Could you check a few things on this model? Use its own coordinates, in mm. Face numbers are marked on the shaded views. A direction names the side the tool comes from. Round coordinates to 2 decimals unless told otherwise and drop trailing zeros. Order: outer loops, then holes, each group sorted by start corner. A loop starts at its lowest first (then second) coordinate and runs counter-clockwise, first axis right, second up.
```python
from build123d import *

# Parameters (mm, degrees)
F2_R = 0.25
F3_R = 0.5
F4_R = 0.25


with BuildPart() as f1:
    # F0 (on Right) → F1 (revolve)
    with BuildSketch(Plane.YZ):
        Polygon((4, 6.35), (2.5, 6.35), (2.5, -2.5), (3.7, -2.5), (3.7, 0), (5.42, 0), (5.42, 2), (4, 2), align=None)
    revolve(axis=Axis((0, 0, -1.722812), (0, 0, -1)))

    # F2
    f2_edges = [f1.edges().sort_by_distance(p)[0] for p in [
        (0, -2.5, 6.35),
    ]]
    fillet(f2_edges, radius=F2_R)

    # F3
    f3_edges = [f1.edges().sort_by_distance(p)[0] for p in [
        (0, -4, 6.35),
    ]]
    fillet(f3_edges, radius=F3_R)

    # F4
    f4_edges = [f1.edges().sort_by_distance(p)[0] for p in [
        (0, -5.42, 2),
    ]]
    fillet(f4_edges, radius=F4_R)


solid = f1.part
```
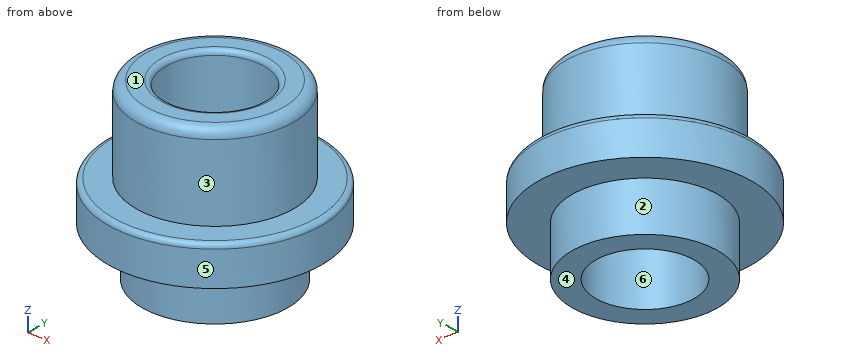
Q1. I need wall thicknesses on L1, parallel to X at y = 0, z = 4.25; L2, parallel to X at y = 0, z = 0.25; L3, parallel to Z at x = -1, y = -4.5. Which ranges of each line are inside material? Lowest first, please.
Q2. We'd pull the mould along Y, two halves only. Please class the marked faces 4, 5 and 6: released by +Y, released by -Y, zero draft, split by the parting line, or undercut.
Q3. Imagine slicing it at A-A, the plane x = 0. Please give me the cut outline in (y, z).
Q4. For P1, Ø6.5, axis at x = 0, y = 0, coming from the +Z side; P2, Ø4, axis at x = -3.5, z = 5, coming from the +Y side; P3, Ø4, axis at x = -4, z = 4.5, coming from the -Y side; P4, Ø1, axis at x = -3, z = 4, coming from the +Y side, each with a flat end and sliding along its axis, tell me the tip position at first contact or that it passes through.
Q5. Imagine slicing it at C-C, the plane z = 0.75. Please give me the cut outline in (x, y), then the cut area to 3 significant figures.
Q6. Imagine slicing it at D-D, the plane z = 3. Please give me the cut outline in (x, y).
Q7. For the marked faces 1, 2 and 3, which set-ups out of +Z, -Z, +X, -X, +Y, -Y let a thin tool reach every point of the face, with its end or its side?
Filled in:
1. L1: x = -4 to -2.5, 2.5 to 4
1. L2: x = -5.42 to -2.5, 2.5 to 5.42
1. L3: z = 0 to 2
2. face 4: zero draft
2. face 5: split by the parting line
2. face 6: undercut
3. outline: (-5.42, 0) - (-3.7, 0) - (-3.7, -2.5) - (-2.5, -2.5) - (-2.5, 6.1) arc R0.25 ccw to (-2.75, 6.35) - (-3.5, 6.35) arc R0.5 ccw to (-4, 5.85) - (-4, 2) - (-5.17, 2) arc R0.25 ccw to (-5.42, 1.75) - close; (2.5, -2.5) - (3.7, -2.5) - (3.7, 0) - (5.42, 0) - (5.42, 1.75) arc R0.25 ccw to (5.17, 2) - (4, 2) - (4, 5.85) arc R0.5 ccw to (3.5, 6.35) - (2.75, 6.35) arc R0.25 ccw to (2.5, 6.1) - close
4. P1: stops at z = 6.35
4. P2: stops at y = 3.71
4. P3: stops at y = -3.46
4. P4: stops at y = 3.12
5. outline: circle Ø10.84 at (0, 0); hole circle Ø5 at (0, 0)
5. area: 72.7 mm2
6. outline: circle Ø8 at (0, 0); hole circle Ø5 at (0, 0)
7. face 1: +Z, +X, -X, +Y, -Y
7. face 2: -Z
7. face 3: +Z
